Print and shaded views of the part. All mm, measured from the part's lowest x, y and z. A direction names the side the tool comes from. Give positions to 0.01 mm unless a question says otherwise; leave off trailing zeros. Order: outer loops, then holes, each group sorted by start corner. A loop starts at its lowest first (then second) coordinate and runs counter-clockwise, first axis right, second up. Notation, with made-up numbers: (7, 76.5) - (60, 76.5) arc R15 ccw to (60, 88.5) - close; hole circle Ø2 at (62, 81.25). An arc over 180 degrees is marked (long way). Answer in a Markdown table with one row per item.
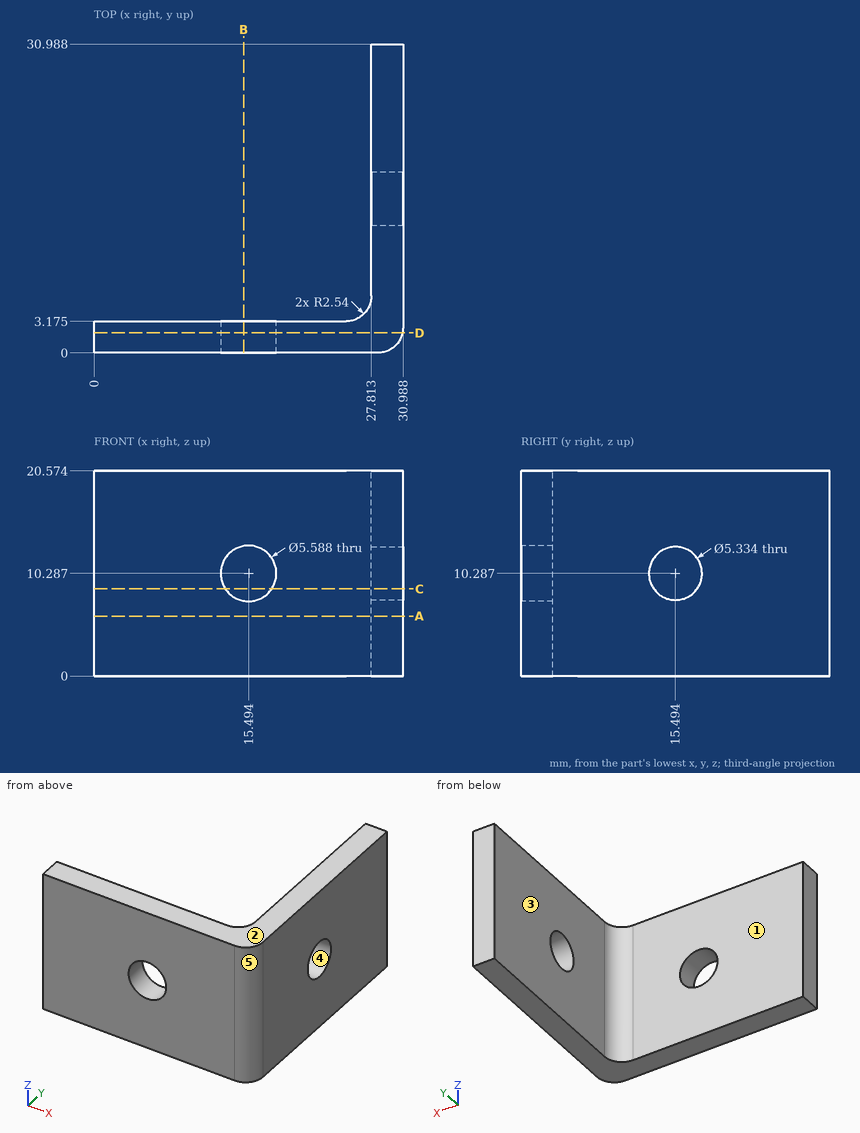
1. Cut at D-D on y = 2. Write the cut outline in (x, z).
Check result:
| item | result |
|---|---|
| outline | (0, 0) - (30.93, 0) - (30.93, 20.57) - (0, 20.57) - close; hole circle Ø5.59 at (15.49, 10.29) |
2. Cut at B-B on x = 15. Write the cut outline in (y, z) (3 decimals), and give its area (3 significant figures).
Check result:
| item | result |
|---|---|
| outline | (0, 0) - (3.175, 0) - (3.175, 7.537) - (0, 7.537) - close; (0, 13.037) - (3.175, 13.037) - (3.175, 20.574) - (0, 20.574) - close |
| area | 47.9 mm² |
3. Two-plate mould, pull along Y, no slides. Class the marked faces 3, 4 and 5: +Y half, -Y half, draft (parallel to the pull), parting line (faces both ways), or undercut.
Check result:
| item | result |
|---|---|
| face 3 | draft |
| face 4 | undercut |
| face 5 | -Y half |
4. Probe line 1 (X direction, y = 15.5, z = 13.5); line 2 (Y direction, x = 4.5, z = 3.25) (3 decimals); line 3 (Y direction, x = 29, z = 14). List the from-to ranges inside material, lowest first.
Check result:
| item | result |
|---|---|
| line 1 | x = 27.81 to 30.99 |
| line 2 | y = 0 to 3.175 |
| line 3 | y = 0.06 to 30.99 |
5. Cut at C-C on z = 8.75. Write the cut outline in (x, y) (3 decimals).
Check result:
| item | result |
|---|---|
| outline | (0, 0) - (13.161, 0) - (13.161, 3.175) - (0, 3.175) - close; (17.827, 0) - (28.448, 0) arc R2.54 ccw to (30.988, 2.54) - (30.988, 13.314) - (27.813, 13.314) - (27.813, 5.715) arc R2.54 cw to (25.273, 3.175) - (17.827, 3.175) - close; (27.813, 17.674) - (30.988, 17.674) - (30.988, 30.988) - (27.813, 30.988) - close |
6. Cut at A-A on z = 6. Write the cut outline in (x, y) (3 decimals).
Check result:
| item | result |
|---|---|
| outline | (0, 0) - (28.448, 0) arc R2.54 ccw to (30.988, 2.54) - (30.988, 30.988) - (27.813, 30.988) - (27.813, 5.715) arc R2.54 cw to (25.273, 3.175) - (0, 3.175) - close |
7. Drop flat-ended pins along their axis: P1, Ø5, axis at y = 15.494, z = 10.287, coming from the +X side; P2, Ø3, axis at x = 5.5, z = 7, coming from the -Y side; P3, Ø10, axis at y = 27.5, z = 5.5, coming from the -X side; P4, Ø4, axis at x = 5, z = 6, coming from the +Y side (3 decimals). Give the stop position or say it passes through.
Check result:
| item | result |
|---|---|
| P1 | passes through |
| P2 | stops at y = 0 |
| P3 | stops at x = 27.81 |
| P4 | stops at y = 3.175 |
8. Which spindle directions (+Z, -Z, +X, -X, +Y, -Y) get a long thin tool onto all of the face, cutting with end or side? Do the marked faces 1 and 2. Say none if no direction does.
Check result:
| item | result |
|---|---|
| face 1 | +Z, -Z, -X, +Y |
| face 2 | +Z, +X, -X, +Y, -Y |
